Check sheet for the modelled part. Datum: model origin and axes. Units: mm. Round coordinates to 2 decimals unless told otherwise and drop trailing zeros. Write each loop counter-clockwise with the first axis right and the second up, starting at its lowest first coordinate (ties: lowest second). Pieces come first, ordered by that corner, then holes.
Item 1: Material ranges on line 1 along Y through (x, z) = (0, 366); line 2 along X through (y, z) = (-1.5, 323); line 3 along X through (y, z) = (50, 175.5), recorded low to high.
Item 2: Depth check by flat-ended pin: pin 1 (4 mm diameter, centred on y = 16.5, z = 340.5, fed in from +X); pin 2 (4 mm diameter, centred on x = -52, z = 219.5, fed in from -Y); pin 3 (6 mm diameter, centred on x = -40, z = 284.5, fed in from -Y). Enter the tip coordinate at first touch or a pass-through.
Item 3: Release check for a two-part mould opening along X. For faces 1 (the flat face through (-62.4, 39.9, 0)), 2 (the cylindrical face through (-16.513, -74.363, 200.355)), 3 (the cylindrical face through (-9.622, 73.285, 262.966)) record: pulls with the +X half, pulls with the -X half, needs draft (parallel to the pull), parting line crosses it, or undercut.
Item 4: Section check C-C, the plane z = 239. Record the cut outline in (x, y) (3 decimals), plus the area to 3 significant figures.
Item 5: Section check D-D, the plane z = 370. Record the cut outline in (x, y).
from build123d import *

# Parameters (mm, degrees)
ESQUISSE2_R                  = 76.1746
ESQUISSE2_R_2                = 73.914
BOSS_EXTRU_1_DEPTH           = 406.4
ESQUISSE3_R                  = 76.2
ESQUISSE3_R_2                = 73.914
BOSS_EXTRU_2_DEPTH           = 127
ESQUISSE4_W                  = 6.35
ESQUISSE4_H                  = 254
ENL_V_MAT_EXTRU_1_DEPTH      = 96.774
R_P_TITION_CIRCULAIRE1_COUNT = 3


with BuildPart() as part:
    # Esquisse2 → Boss.-Extru.1 (new body)
    with BuildSketch(Plane.XY):
        Circle(ESQUISSE2_R)
        Circle(ESQUISSE2_R_2, mode=Mode.SUBTRACT)
    extrude(amount=BOSS_EXTRU_1_DEPTH)

    # Esquisse3 → Boss.-Extru.2 (add)
    with BuildSketch(Plane.XY.offset(406.4)):
        Circle(ESQUISSE3_R)
        Circle(ESQUISSE3_R_2, mode=Mode.SUBTRACT)
    extrude(amount=BOSS_EXTRU_2_DEPTH)

    # Esquisse4 → Enlèv. mat.-Extru.1 (cut)
    with BuildSketch(Plane(origin=(0, 0, 0), x_dir=(1, 0, 0), z_dir=(0, 1, 0))):
        with Locations((0, -203.2)):
            Rectangle(ESQUISSE4_W, ESQUISSE4_H)
    enl_v_mat_extru_1 = extrude(amount=ENL_V_MAT_EXTRU_1_DEPTH, mode=Mode.SUBTRACT)

    # Répétition circulaire1: Enlèv. mat.-Extru.1 ×3 about axis
    r_p_tition_circulaire1_axis = Axis((0, 0, 0), (0, 0, 1))
    for i in range(1, R_P_TITION_CIRCULAIRE1_COUNT):
        add(enl_v_mat_extru_1.rotate(r_p_tition_circulaire1_axis, i * 360 / R_P_TITION_CIRCULAIRE1_COUNT), mode=Mode.SUBTRACT)


solid = part.part
Values found:
1. line 1: y = -76.17 to -73.91, 73.91 to 76.17
1. line 2: x = -76.16 to -73.9, 73.9 to 76.16
1. line 3: x = -57.47 to -54.44, 54.44 to 57.47
2. pin 1: stops at x = 74.78
2. pin 2: stops at y = -57.47
2. pin 3: stops at y = -66.59
3. face 1: needs draft
3. face 2: parting line crosses it
3. face 3: undercut
4. outline: (-67.499, -35.305) - (-65.54, -34.173) arc R73.914 cw to (-3.175, 73.846) - (-3.175, 76.108) arc R76.175 ccw to start; (-64.324, -40.804) arc R76.175 ccw to (64.324, -40.804) - (62.365, -39.673) arc R73.914 cw to (-62.365, -39.673) - close; (3.175, 73.846) arc R73.914 cw to (65.54, -34.173) - (67.499, -35.305) arc R76.175 ccw to (3.175, 76.108) - close
4. area: 1,020 mm2
5. outline: circle Ø152.35 at (0, 0); hole circle Ø147.83 at (0, 0)
